from build123d import *

# Parameters (mm, degrees)
SKETCH_W      = 120
SKETCH_H      = 65
PAD_DEPTH     = 1
SKETCH001_W   = 120
SKETCH001_H   = 65
SKETCH001_W_2 = 110
SKETCH001_H_2 = 55
PAD001_DEPTH  = 1.5
SKETCH002_W   = 104
SKETCH002_H   = 49
POCKET_DEPTH  = 1.001
FILLET_R      = 2
FILLET001_R   = 0.9


with BuildPart() as part:
    # Sketch → Pad (new body)
    with BuildSketch(Plane.XY):
        Rectangle(SKETCH_W, SKETCH_H)
    extrude(amount=PAD_DEPTH)

    # Sketch001 (on Face6 of Pad) → Pad001 (join)
    with BuildSketch(Plane.XY.offset(1)):
        Rectangle(SKETCH001_W, SKETCH001_H)
        Rectangle(SKETCH001_W_2, SKETCH001_H_2, mode=Mode.SUBTRACT)
    extrude(amount=PAD001_DEPTH)

    # Sketch002 (on Face15 of Pad001) → Pocket (cut, through all)
    with BuildSketch(Plane.XY.offset(1)):
        Rectangle(SKETCH002_W, SKETCH002_H)
    extrude(amount=-POCKET_DEPTH, mode=Mode.SUBTRACT)

    # Fillet
    fillet_edges = [part.edges().sort_by_distance(p)[0] for p in [
        (-60, -32.5, 1.75),
        (-60, -32.5, 0.5),
        (60, -32.5, 1.75),
        (60, -32.5, 0.5),
        (-60, 32.5, 1.75),
        (-60, 32.5, 0.5),
        (60, 32.5, 1.75),
        (60, 32.5, 0.5),
    ]]
    fillet(fillet_edges, radius=FILLET_R)

    # Fillet001
    fillet001_edges = [part.edges().sort_by_distance(p)[0] for p in [
        (0, -32.5, 0),
        (0, -24.5, 0),
        (52, 0, 0),
        (0, 24.5, 0),
        (-52, 0, 0),
        (-60, 0, 0),
        (0, 32.5, 0),
        (60, 0, 0),
    ]]
    fillet(fillet001_edges, radius=FILLET001_R)


solid = part.part
The listing builds one solid part. Answer for the finished solid, in the listing's coordinates (mm). Coordinates: 2 decimals unless noted, no trailing zeros. Order: outer loops, then holes, each group sorted by start corner. A loop starts at its lowest first (then second) coordinate and runs counter-clockwise, first axis right, second up.
Q1. For a pull along Y with two mould halves and no side action, classify faces 1 (the face through (0, 25, 1)), 2 (the face through (-5, -29, 2.5)) as pulls with the +Y half, pulls with the -Y half, needs draft (parallel to the pull), parting line crosses it, or undercut.
Q2. A cutting plane is placed at A-A, the plane z = 1.6. Write down the section's boundary in (x, y), and give its area (3 significant figures).
Q3. Consider line 1 (Y direction, x = -20.5, z = 0.7); line 2 (X direction, y = 21.5, z = 1.5); line 3 (Y direction, x = -18.5, z = 1.75). Determine where each line is inside the solid, lowest interval first.
Q4. A cutting plane is placed at B-B, the plane x = 5.5. Write down the section's boundary in (y, z).
Q5. A cutting plane is placed at C-C, the plane y = 8.5. Write down the section's boundary in (x, z).
Answers follow:
1. face 1: undercut
1. face 2: needs draft
2. outline: (-60, -30.5) arc R2 ccw to (-58, -32.5) - (58, -32.5) arc R2 ccw to (60, -30.5) - (60, 30.5) arc R2 ccw to (58, 32.5) - (-58, 32.5) arc R2 ccw to (-60, 30.5) - close; hole (-55, -27.5) - (55, -27.5) - (55, 27.5) - (-55, 27.5) - close
2. area: 1,750 mm2
3. line 1: y = -32.48 to -24.52, 24.52 to 32.48
3. line 2: x = -60 to -55, 55 to 60
3. line 3: y = -32.5 to -27.5, 27.5 to 32.5
4. outline: (-32.5, 0.9) arc R0.9 ccw to (-31.6, 0) - (-25.4, 0) arc R0.9 ccw to (-24.5, 0.9) - (-24.5, 1) - (-27.5, 1) - (-27.5, 2.5) - (-32.5, 2.5) - close; (24.5, 0.9) arc R0.9 ccw to (25.4, 0) - (31.6, 0) arc R0.9 ccw to (32.5, 0.9) - (32.5, 2.5) - (27.5, 2.5) - (27.5, 1) - (24.5, 1) - close
5. outline: (-60, 0.9) arc R0.9 ccw to (-59.1, 0) - (-52.9, 0) arc R0.9 ccw to (-52, 0.9) - (-52, 1) - (-55, 1) - (-55, 2.5) - (-60, 2.5) - close; (52, 0.9) arc R0.9 ccw to (52.9, 0) - (59.1, 0) arc R0.9 ccw to (60, 0.9) - (60, 2.5) - (55, 2.5) - (55, 1) - (52, 1) - close
